Part model, mm, in its own coordinate system. Face numbers are marked on the shaded views. A direction names the side the tool comes from. Give positions to 0.01 mm unless a question says otherwise; leave off trailing zeros. Order: outer loops, then holes, each group sorted by start corner. A loop starts at its lowest first (then second) coordinate and runs counter-clockwise, first axis right, second up. Notation, with made-up numbers: M 68.25,32.25 L 112.25,32.25 A35 cw 112.25,70.25 Z; hole C -4,4.25 d2. An arc over 180 degrees is marked long. Answer as a JSON object with one key per item and string values.
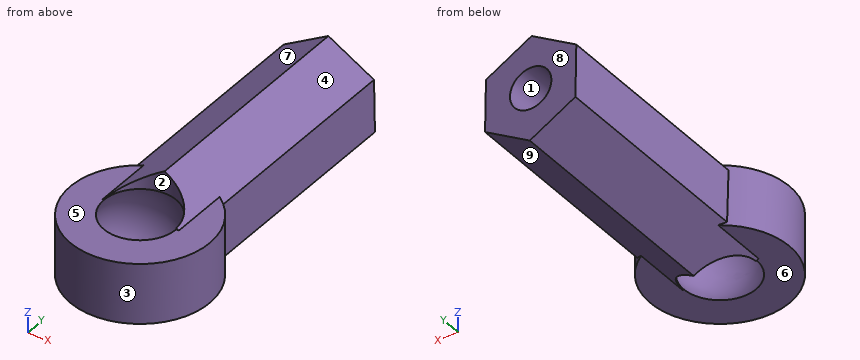
from build123d import *

# Parameters (mm, degrees)
SKETCH_1_R               = 3.7
EXTRUDE_1_DEPTH          = 1.6
EXTRUDE_1_DEPTH_BACK     = 1.6
EXTRUDE_3_DEPTH          = 14.3
SKETCH_9_R               = 1.1
CUT_EXTRUDE_1_DEPTH      = 5
SKETCH_10_R              = 1.920937271
CUT_EXTRUDE_2_DEPTH      = 2.170853659
CUT_EXTRUDE_2_DEPTH_BACK = 5.370853659


with BuildPart() as part:
    # Sketch 1 → Extrude 1 (new body, two sides)
    with BuildSketch(Plane.XY) as extrude_1_sk:
        Circle(SKETCH_1_R)
    extrude(amount=EXTRUDE_1_DEPTH)
    extrude(extrude_1_sk.sketch, amount=-EXTRUDE_1_DEPTH_BACK)

    # Sketch 8 → Extrude 3 (add)
    with BuildSketch(Plane(origin=(0, 0, 0), x_dir=(1, 0, 0), z_dir=(0, 1, 0))):
        Polygon((0.048682641, 2.770853659), (-2.375288338, 1.427587234), (-2.42397098, -1.343266426), (-0.048682641, -2.770853659), (2.375288338, -1.427587234), (2.42397098, 1.343266426), align=None)
    extrude(amount=EXTRUDE_3_DEPTH)

    # Sketch 7 → Cut-Revolve 7 (revolve, cut)
    with BuildSketch(Plane.XY):
        with BuildLine():
            Line((0, 2.5), (0, -2.5))
            ThreePointArc((0, -2.5), (2.5, 0), (0, 2.5))
        make_face()
    revolve(axis=Axis((0, 2.5, 0), (0, -1, 0)), mode=Mode.SUBTRACT)

    # Sketch 9 → Cut-Extrude 1 (cut)
    with BuildSketch(Plane(origin=(0, 14.3, 0), x_dir=(1, 0, 0), z_dir=(0, 1, 0))):
        Circle(SKETCH_9_R)
    extrude(amount=-CUT_EXTRUDE_1_DEPTH, mode=Mode.SUBTRACT)

    # Sketch 10 → Cut-Extrude 2 (cut, two sides)
    with BuildSketch(Plane(origin=(0, 0, -1.6), x_dir=(-1, 0, 0), z_dir=(0, 0, -1))) as cut_extrude_2_sk:
        Circle(SKETCH_10_R)
    extrude(amount=CUT_EXTRUDE_2_DEPTH, mode=Mode.SUBTRACT)
    extrude(cut_extrude_2_sk.sketch, amount=-CUT_EXTRUDE_2_DEPTH_BACK, mode=Mode.SUBTRACT)


solid = part.part
1. Cut at D-D on z = 0.2. Give the cut face in (x, y).
Worked answers:
{"outline": "M -2.4,2.81 A3.7 ccw long 2.4,2.82 L 2.4,14.3 L 1.08,14.3 L 1.08,9.3 L -1.08,9.3 L -1.08,14.3 L -2.4,14.3 Z; hole C 0,0 d4.98"}
2. Cut at A-A on y = 1.5. Give the cut face in (x, z).
Worked answers:
{"outline": "M -3.38,-1.6 L -2.06,-1.6 L -1.2,-2.08 L -1.2,-1.6 A2 cw -1.2,1.6 L -1.2,2.08 L -2,1.6 L -3.38,1.6 Z; M 1.2,-2.08 L 2,-1.6 L 3.38,-1.6 L 3.38,1.6 L 2.06,1.6 L 1.2,2.08 L 1.2,1.6 A2 cw 1.2,-1.6 Z"}
3. Two-plate mould, pull along X, no slides. Class the marked faces 1, 2, 3 and 4: +X half, -X half, draft (parallel to the pull), parting line (faces both ways), or undercut.
Worked answers:
{"face 1": "undercut", "face 2": "undercut", "face 3": "parting line", "face 4": "+X half"}
4. Probe line 1 along X through (y, z) = (11.1, 0); line 2 along Y through (x, z) = (0, 0.15); line 3 along Z through (x, y) = (0, 12.4). List the from-to ranges inside material, lowest first.
Worked answers:
{"line 1": "x = -2.4 to -1.1, 1.1 to 2.4", "line 2": "y = -3.7 to -2.5, 2.5 to 9.3", "line 3": "z = -2.74 to -1.1, 1.1 to 2.74"}
5. Cut at C-C on y = 10.5. Give the cut face in (x, z).
Worked answers:
{"outline": "M -2.42,1.34 L -2.38,-1.43 L 0.05,-2.77 L 2.42,-1.34 L 2.38,1.43 L -0.05,2.77 Z; hole C 0,0 d2.2"}
6. Pin check, flat tips, straight feed: P1, Ø2, axis at y = -1.5, z = -0.5, coming from the +X side; P2, Ø1, axis at x = 3, y = 12, coming from the +Z side. Stop position of each tip, or through.
Worked answers:
{"P1": "stops at x = 3.67", "P2": "passes through"}
7. Which spindle directions (+Z, -Z, +X, -X, +Y, -Y) get a long thin tool onto all of the face, cutting with end or side? Do the marked faces 5, 6, 7, 8 and 9. Say none if no direction does.
Worked answers:
{"face 5": "+Z, -Y", "face 6": "-Z, -Y", "face 7": "+Z, -X, +Y", "face 8": "+Z, -Z, +X, -X, +Y", "face 9": "-Z, +X, +Y"}
8. Cut at B-B on x = 1.75. Give the cut face in (y, z).
Worked answers:
{"outline": "M -3.26,-1.6 L -0.79,-1.6 A1.79 cw -0.79,1.6 L -3.26,1.6 Z; M 0.79,-1.75 L 14.3,-1.75 L 14.3,1.77 L 0.79,1.77 L 0.79,1.6 A1.79 cw 0.79,-1.6 Z"}
